Check sheet for the modelled part. Datum: model origin and axes. Units: mm. Face numbers are marked on the shaded views. A direction names the side the tool comes from. Round coordinates to 2 decimals unless told otherwise and drop trailing zeros. Write each loop counter-clockwise with the first axis right and the second up, starting at its lowest first coordinate (ties: lowest second). Pieces come first, ordered by that corner, then holes. Notation, with made-up numbers: (87.5, 11) -> (101.5, 11) arc R26 ccw to (101.5, 28) -> close; hole circle Ø3 at (-34, 9.5). An arc over 180 degrees is marked (long way). Answer as a JSON object with one key per item and string values. Group by question number.
```python
from build123d import *

# Parameters (mm, degrees)
SKETCH1_W                  = 4.4
SKETCH1_H                  = 10
BOSS_EXTRUDE1_DEPTH        = 10
SKETCH2_R                  = 1.5
BOSS_EXTRUDE2_DEPTH        = 1.5
DOME1_FACE_RADIUS          = 1.5
DOME1_HEIGHT               = 1
MIRROR1_COPY_1_FACE_RADIUS = 1.5
MIRROR1_COPY_1_HEIGHT      = 1


with BuildPart() as part:
    # Sketch1 → Boss-Extrude1 (new body)
    with BuildSketch(Plane.XY):
        Rectangle(SKETCH1_W, SKETCH1_H)
    extrude(amount=-BOSS_EXTRUDE1_DEPTH)

    # Sketch2 → Boss-Extrude2 (add)
    with BuildSketch(Plane.XY):
        with Locations((0, 2.5)):
            Circle(SKETCH2_R)
    boss_extrude2 = extrude(amount=BOSS_EXTRUDE2_DEPTH)

    # Dome1: a dome of height H over a round flat face of radius A is a cap of a sphere of radius (A * A + H * H) / (2 * H)
    dome1_r = (DOME1_FACE_RADIUS * DOME1_FACE_RADIUS + DOME1_HEIGHT * DOME1_HEIGHT) / (2 * DOME1_HEIGHT)
    dome1_base = Plane((0, 2.5, 1.5), z_dir=(0, 0, 1))
    with Locations(dome1_base.offset(DOME1_HEIGHT - dome1_r)):
        dome1_ball = Sphere(dome1_r, mode=Mode.PRIVATE)
    add(split(dome1_ball, bisect_by=dome1_base, keep=Keep.TOP, mode=Mode.PRIVATE))

    # Mirror1: Boss-Extrude2 across plane
    add(boss_extrude2.mirror(Plane.ZX))

    # Mirror1 copy 1: a dome of height H over a round flat face of radius A is a cap of a sphere of radius (A * A + H * H) / (2 * H)
    mirror1_copy_1_r = (MIRROR1_COPY_1_FACE_RADIUS * MIRROR1_COPY_1_FACE_RADIUS + MIRROR1_COPY_1_HEIGHT * MIRROR1_COPY_1_HEIGHT) / (2 * MIRROR1_COPY_1_HEIGHT)
    mirror1_copy_1_base = Plane((0, -2.5, 1.5), z_dir=(0, 0, 1))
    with Locations(mirror1_copy_1_base.offset(MIRROR1_COPY_1_HEIGHT - mirror1_copy_1_r)):
        mirror1_copy_1_ball = Sphere(mirror1_copy_1_r, mode=Mode.PRIVATE)
    add(split(mirror1_copy_1_ball, bisect_by=mirror1_copy_1_base, keep=Keep.TOP, mode=Mode.PRIVATE))


solid = part.part
```
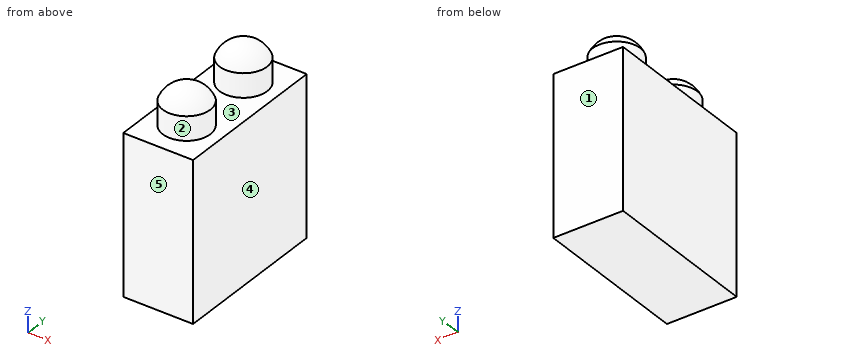
(1) Release check for a two-part mould opening along Y. For the marked faces 3, 4 and 5 record: pulls with the +Y half, pulls with the -Y half, needs draft (parallel to the pull), parting line crosses it, or undercut.
(2) Scan lines: line 1 along Y through (x, z) = (-0.8, 1.75); line 2 along Z through (x, y) = (2, -1.5); line 3 along Z through (x, y) = (0.75, -2). Record each from-to range of solid material in increasing order.
(3) Section check C-C on x = 0. Record the cut outline in (y, z) (3 decimals).
(4) Section check A-A on x = -0.9. Record the cut outline in (y, z) (3 decimals), then the cut area to 3 significant figures.
(5) Section check D-D on y = 3.25. Record the cut outline in (x, z) (3 decimals).
(6) Access from +Z, -Z, +X, -X, +Y, -Y to the whole of each face (thin tool, end or side, straight path). Record for the marked faces 1 and 2.
(7) Section check B-B on y = -2.5. Record the cut outline in (x, z) (3 decimals), then the cut area to 3 significant figures.
(8) Go/stop test with a flat-tipped pin: pin 1 Ø2 at (x, y) = (1, -0.5) entering from +Z. Record where the tip stops, or that it passes through.
Data:
{
 "1": {"face 3": "undercut", "face 4": "needs draft", "face 5": "pulls with the -Y half"},
 "2": {"line 1": "y = -3.61 to -1.39, 1.39 to 3.61", "line 2": "z = -10 to 0", "line 3": "z = -10 to 2.23"},
 "3": {"outline": "(-5, -10) -> (5, -10) -> (5, 0) -> (4, 0) -> (4, 1.5) arc R1.625 ccw to (1, 1.5) -> (1, 0) -> (-1, 0) -> (-1, 1.5) arc R1.625 ccw to (-4, 1.5) -> (-4, 0) -> (-5, 0) -> close"},
 "4": {"outline": "(-5, -10) -> (5, -10) -> (5, 0) -> (3.7, 0) -> (3.7, 1.5) arc R1.353 ccw to (1.3, 1.5) -> (1.3, 0) -> (-1.3, 0) -> (-1.3, 1.5) arc R1.353 ccw to (-3.7, 1.5) -> (-3.7, 0) -> (-5, 0) -> close", "area": "110 mm²"},
 "5": {"outline": "(-2.2, -10) -> (2.2, -10) -> (2.2, 0) -> (1.299, 0) -> (1.299, 1.5) arc R1.442 ccw to (-1.299, 1.5) -> (-1.299, 0) -> (-2.2, 0) -> close"},
 "6": {"face 1": "+Z, -Z, +X, -X, +Y", "face 2": "+Z"},
 "7": {"outline": "(-2.2, -10) -> (2.2, -10) -> (2.2, 0) -> (1.5, 0) -> (1.5, 1.5) arc R1.625 ccw to (-1.5, 1.5) -> (-1.5, 0) -> (-2.2, 0) -> close", "area": "50.7 mm²"},
 "8": {"pin 1": "stops at z = 1.93"}
}
